Drawing for the job (mm, zero at the part's lowest x, y, z). Give positions to 0.01 mm unless a question says otherwise; leave off trailing zeros. Write each loop counter-clockwise with the first axis right and the second up, starting at its lowest first coordinate (ties: lowest second). Pieces come first, ordered by that corner, then holes. Notation, with made-up numbers: (-4, 87) - (45, 87) arc R28 ccw to (45, 108) - close; hole circle Ø10 at (3.25, 47.25). An arc over 180 degrees is marked (long way). Use CSV: the item, a comma, the result in double quotes.
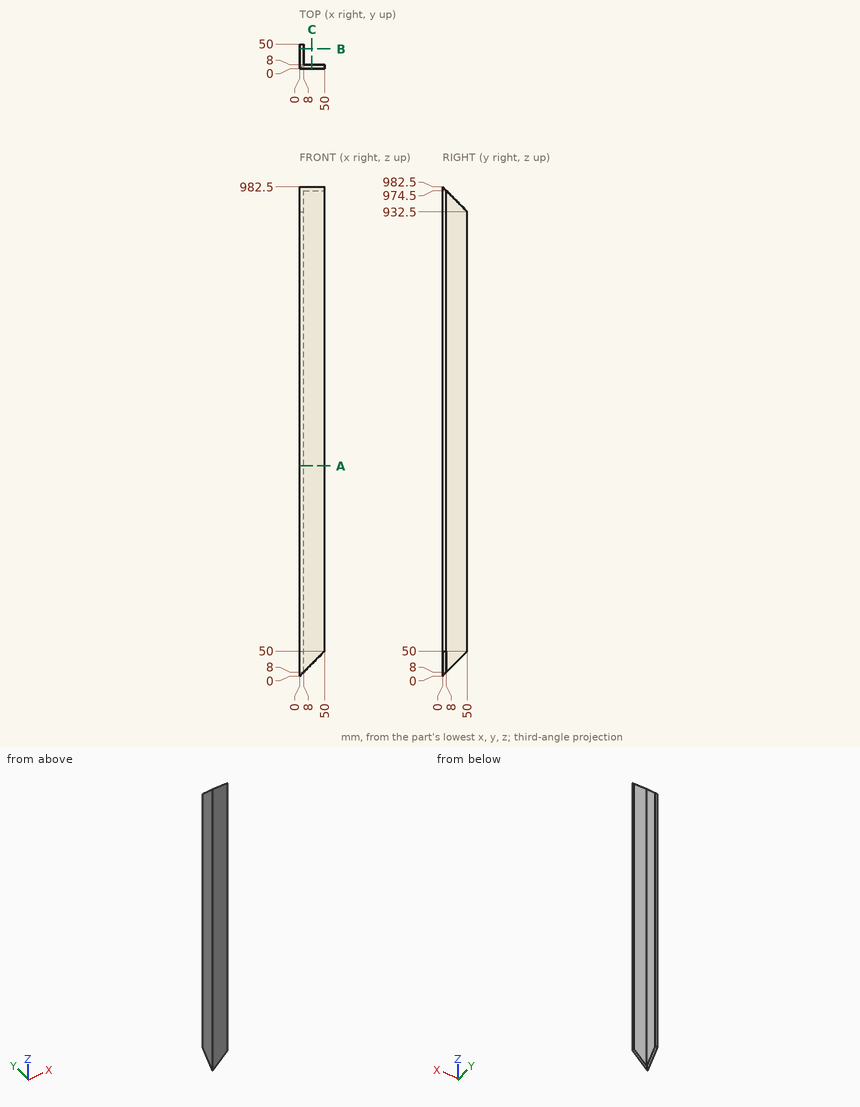
(1) Wall check: probe 1 along X at (y, z) = (25, 430); probe 2 along Z at (x, y) = (3.5, 30). Give the ranges that are in metal, low to high. Write a range as [from, to].
Checked values:
probe 1,"x = [0, 8]"
probe 2,"z = [30, 952.5]"
(2) Saw through at A-A, the plane z = 422. List the corners of the cut face in (x, y).
Checked values:
outline,"(0, 0) - (50, 0) - (50, 8) - (8, 8) - (8, 50) - (0, 50) - close"
(3) Flat gauge pins, fed straight in: P1, Ø1.5, axis at y = 39.5, z = 501, coming from the +X side; P2, Ø1, axis at x = 24.5, z = 544.5, coming from the +Y side. Where does each tip first touch, or does it go through?
Checked values:
P1,"stops at x = 8"
P2,"stops at y = 8"
(4) Saw through at B-B, the plane y = 40. List the corners of the cut face in (x, z).
Checked values:
outline,"(0, 40) - (8, 40) - (8, 942.5) - (0, 942.5) - close"
(5) Saw through at C-C, the plane x = 24.5. List the corners of the cut face in (y, z).
Checked values:
outline,"(0, 24.5) - (8, 24.5) - (8, 974.5) - (0, 982.5) - close"
